Autodesk Fusion 360 part; units mm, degrees
sketch "Sketch1" plane through (0, 0, 0) normal (0, 1, 0) x (1, 0, 0)
  line L0 (0, 0) -> (59, 0)
  line L1 (59, 0) -> (59, 54)
  line L2 (59, 54) -> (0, 54)
  line L3 (0, 54) -> (0, 0)
  dimension "d1" = 59
  dimension "d2" = 54
extrude "Extrude1" add sketch "Sketch1" along normal blind 3 makes body 1
sketch "Sketch2" plane through (0, 3, 0) normal (0, 1, 0) x (-1, 0, 0)
  line L0 (0, -54) -> (0, 0)
  line L1 (0, 0) -> (-59, 0)
  line L2 (-59, 0) -> (-59, -54)
  line L3 (-59, -54) -> (0, -54)
  line L4 (-57, -2) -> (-2, -2)
  line L5 (-2, -2) -> (-2, -52)
  line L6 (-2, -52) -> (-57, -52)
  line L7 (-57, -52) -> (-57, -2)
  line L8 (-57, -2) -> (-2, -52) construction
  line L9 (-2, -2) -> (-57, -52) construction
  point P0 (-29.5, -27)
  dimension "d5" = 55
  dimension "d6" = 50
  dimension "d15" = 27
  dimension "d16" = 29.5
extrude "Extrude2" add sketch "Sketch2" along normal blind 27 bodies 1
sketch "Sketch3" plane through (59, 0, 0) normal (1, 0, 0) x (0, 0, -1)
  line L0 (0, 0) -> (54, 0)
  line L1 (54, 0) -> (54, 30)
  line L2 (54, 30) -> (0, 30)
  line L3 (0, 30) -> (0, 0)
  line L4 (12, 25) -> (32, 25)
  line L5 (32, 25) -> (32, 15)
  line L6 (32, 15) -> (12, 15)
  line L7 (12, 15) -> (12, 25)
  dimension "d9" = 20
  dimension "d10" = 10
  dimension "d11" = 12
  dimension "d12" = 15
extrude "Extrude3" cut sketch "Sketch3" against normal blind 3 contours L4 L5 L6 L7 bodies 1
sketch "Sketch4" plane through (0, 0, 0) normal (-1, 0, 0) x (0, 0, 1)
  line L0 (-54, 0) -> (0, 0)
  line L1 (0, 0) -> (0, 30)
  line L2 (0, 30) -> (-54, 30)
  line L3 (-54, 30) -> (-54, 0)
  line L4 (-50.5, 10) -> (-43.5, 10)
  line L5 (-43.5, 10) -> (-43.5, 7)
  line L6 (-43.5, 7) -> (-50.5, 7)
  line L7 (-50.5, 7) -> (-50.5, 10)
  dimension "d17" = 7
  dimension "d18" = 3
  dimension "d19" = 7
  dimension "d20" = 3.5
extrude "Extrude4" cut sketch "Sketch4" against normal blind 4 contours L4 L5 L6 L7 bodies 1
sketch "Sketch11" plane through (0, 0, 0) normal (1, 0, 0) x (0, 0, -1)
  circle A0 centre (27, -16) radius 12.11
  line L0 (0, 0) -> (54, 0)
  line L1 (7, 0) -> (47, 0)
  line L2 (47, 0) -> (47, -16)
  line L3 (47, -16) -> (7, -16)
  line L4 (7, -16) -> (7, 0)
  line L5 (54, 0) -> (54, 30)
  dimension "d55" = 24.22
  dimension "d57" = 16
  dimension "d60" = 40
  dimension "d65" = 7
  dimension "d67" = 16
extrude "Extrude9" add sketch "Sketch11" along normal blind 59 separate body contours A0 L0 L1 L2 L3 L4 makes body 2
sketch "Sketch12" plane through (0, 0, 0) normal (0, 1, 0) x (1, 0, 0)
  line L0 (-4, 27) -> (62, 27)
  line L1 (-5, 0) -> (64, 0)
  line L2 (-3, 54) -> (63, 54)
  dimension "d64" = 27
combine "Combine1" operation add target body 2 tool bodies 1
fillet "Fillet1" radius 5 1 edges at (29.5, 0, -7) on bodies 2
fillet "Fillet2" radius 5 1 edges at (29.5, 0, -47) on bodies 2
sketch "Sketch16" plane through (0, -16, 0) normal (0, -1, 0) x (1, 0, 0)
  line L0 (0, -39.11) -> (0, -47)
  line L1 (0, -47) -> (59, -47)
  line L2 (59, -47) -> (59, -39.11)
  line L3 (59, -39.11) -> (0, -39.11)
  line L4 (22, -40.555) -> (10, -40.555)
  line L5 (10, -40.555) -> (10, -43.555)
  line L6 (10, -43.555) -> (22, -43.555)
  line L7 (22, -43.555) -> (22, -40.555)
  line L8 (22, -40.555) -> (10, -43.555) construction
  line L9 (10, -40.555) -> (22, -43.555) construction
  line L10 (37, -40.555) -> (37, -43.555)
  line L11 (49, -43.555) -> (49, -40.555)
  line L12 (37, -40.555) -> (49, -43.555) construction
  line L13 (37, -43.555) -> (49, -43.555)
  line L14 (49, -40.555) -> (37, -40.555)
  line L15 (49, -40.555) -> (37, -43.555) construction
  point P0 (16, -42.055)
  point P1 (43, -42.055)
  dimension "d72" = 12
  dimension "d73" = 3
  dimension "d74" = 4.945
  dimension "d75" = 12
  dimension "d76" = 3
  dimension "d77" = 10
  dimension "d78" = 10
  dimension "d84" = 4.945
revolve "Revolve1" cut sketch "Sketch16" angle 360 about axis through (-4, 0, -27) along (1, 0, 0) contours L4 L5 L6 L7 | L10 L11 L13 L14 bodies 2
fillet "Fillet3" radius 2 1 edges at (29.5, -16, -47) on bodies 2
fillet "Fillet4" radius 2 1 edges at (29.5, -16, -7) on bodies 2
equation "d74 = 4.5 mm + 0.445 mm"
equation "d84 = 4.5 mm + 0.445 mm"
Model file for the job. Use its own axes, mm. A direction names the side the tool comes from. Give positions to 0.01 mm unless a question says otherwise; leave off trailing zeros. Loops run counter-clockwise (first coordinate to the right, second up) from the corner with the lowest first, then second, coordinate; pieces in that order, holes last. Notation, with made-up numbers: (49, 44) -> (64, 44) arc R7 cw to (64, 51) -> close; hole circle Ø6 at (59.25, 27.5). An arc over 180 degrees is marked (long way). Use CSV: the item, a comma, the result in double quotes. Start each with the question number.
1) Flat gauge pins, fed straight in: pin 1 Ø6 at (x, y) = (45, 4.5) entering from +Z; pin 2 Ø1 at (x, z) = (0.5, -46.5) entering from -Y; pin 3 Ø0.6 at (x, z) = (24.5, -1) entering from -Y; pin 4 Ø3 at (x, z) = (36.5, -44) entering from +Y. Where does each tip first touch, or does it go through?
2) Wall check: line 1 (X direction, y = 0.5, z = -48); line 2 (Z direction, x = 16, y = 11.5); line 3 (X direction, y = 16, z = -32.5). Give the ranges that are in metal, low to high.
3) Slice it at C-C on x = 45. Give the number of separate pieces and of enclosed holes in the cut face, plus the area to 3 significant figures.
4) Slice it at A-A on z = -27. Give the cut face in (x, y), plus the area to 3 significant figures.
5) Mould opens along X. For faces 1 (the flat face through (22, -13, -45)), 2 (the flat face through (1, 7, -47)), 3 (the flat face through (49, -13, -9)), 4 (the flat face through (0, 12, -27)) say: released by +X, released by -X, zero draft, split by the parting line, or undercut.
6) Slice it at B-B on y = 16. Give the cut face in (x, z).
7) Slice it at D-D on x = 53. Give the cut face in (y, z).
8) Tool access for faces 5 (the cylindrical face through (42.92, -11.54, -44.51)), 6 (the flat face through (57, 13, -27)), 7 (the flat face through (58, 20, -12)): list every direction of +Z, -Z, +X, -X, +Y, -Y with a clear straight run to the whole face (end or side of a thin tool).
Computed values:
1,pin 1,"stops at z = 0"
1,pin 2,"stops at y = -15.73"
1,pin 3,"stops at y = 0"
1,pin 4,"stops at y = 3"
2,line 1,"x = 0 to 10, 22 to 37, 49 to 59"
2,line 2,"z = -54 to -52, -2 to 0"
2,line 3,"x = 0 to 2, 57 to 59"
3,separate pieces,"5"
3,enclosed holes,"0"
3,area,"637 mm^2"
4,outline,"(0, -3.89) -> (59, -3.89) -> (59, 15) -> (57, 15) -> (57, 3) -> (2, 3) -> (2, 30) -> (0, 30) -> close; (57, 25) -> (59, 25) -> (59, 30) -> (57, 30) -> close"
4,area,"495 mm^2"
5,face 1,"undercut"
5,face 2,"zero draft"
5,face 3,"undercut"
5,face 4,"released by -X"
6,outline,"(0, -54) -> (59, -54) -> (59, -32) -> (57, -32) -> (57, -52) -> (2, -52) -> (2, -2) -> (57, -2) -> (57, -12) -> (59, -12) -> (59, 0) -> (0, 0) -> close"
7,outline,"(-16, -45) arc R2 ccw to (-14, -47) -> (-5, -47) arc R5 cw to (0, -52) -> (0, -54) -> (30, -54) -> (30, -52) -> (3, -52) -> (3, -2) -> (30, -2) -> (30, 0) -> (0, 0) -> (0, -2) arc R5 cw to (-5, -7) -> (-14, -7) arc R2 ccw to (-16, -9) -> (-16, -14.89) arc R12.11 cw to (-16, -39.11) -> close"
8,face 5,"none"
8,face 6,"+Y"
8,face 7,"+X"
